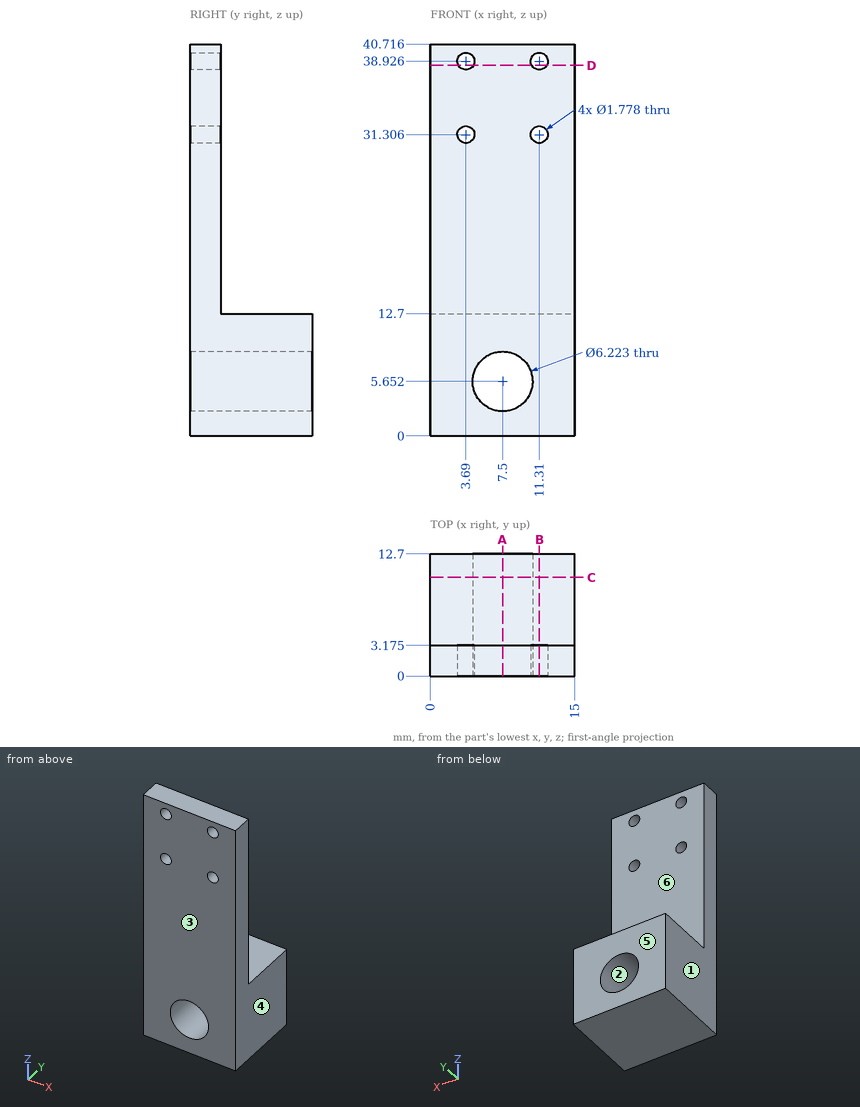
Design review of the part shown in the three views and the two pictorial views. Dimensions are in mm from the part's minimum x, y and z. A direction names the side the tool comes from. Coordinates: 2 decimals unless noted, no trailing zeros. Loops run counter-clockwise (first coordinate to the right, second up) from the corner with the lowest first, then second, coordinate; pieces in that order, holes last. Notation, with made-up numbers: M 26.5,6 L 78.5,6 A27 ccw 78.5,35 Z; hole C 26.5,45 d6. An arc over 180 degrees is marked long. One line per question, with ' | ' between items.
(1) We need section D-D (z = 38.5). Give the boundary of the cut face in (x, y) (1 decimal).
Filled in:
outline: M 0,0 L 2.9,0 L 2.9,3.2 L 0,3.2 Z; M 4.5,0 L 10.5,0 L 10.5,3.2 L 4.5,3.2 Z; M 12.1,0 L 15,0 L 15,3.2 L 12.1,3.2 Z
(2) We need section A-A (x = 7.5). Give the boundary of the cut face in (y, z) (1 decimal), and give its area (3 significant figures).
Filled in:
outline: M 0,0 L 12.7,0 L 12.7,2.5 L 0,2.5 Z; M 0,8.8 L 12.7,8.8 L 12.7,12.7 L 3.2,12.7 L 3.2,40.7 L 0,40.7 Z | area: 171 mm^2
(3) We need section B-B (x = 11.31). Give the boundary of the cut face in (y, z) (1 decimal).
Filled in:
outline: M 0,0 L 12.7,0 L 12.7,12.7 L 3.2,12.7 L 3.2,30.4 L 0,30.4 Z; M 0,32.2 L 3.2,32.2 L 3.2,38 L 0,38 Z; M 0,39.8 L 3.2,39.8 L 3.2,40.7 L 0,40.7 Z
(4) Draft analysis for pull direction X (two halves, no side actions). For the marked faces 1, 2, 3 and 4, state which applies: released by +X, released by -X, zero draft, split by the parting line, or undercut.
Filled in:
face 1: released by -X | face 2: undercut | face 3: zero draft | face 4: released by +X
(5) For pin 1 Ø1.1 at (x, z) = (3.69, 31.31) entering from +Y; pin 2 Ø1.5 at (x, y) = (10.5, 5.5) entering from +Z; pin 3 Ø8 at (x, z) = (8, 29.5) entering from +Y (1 decimal), all flat-tipped, find the tip position at first contact; note any pin that passes through.
Filled in:
pin 1: passes through | pin 2: stops at z = 12.7 | pin 3: stops at y = 3.2
(6) We need section C-C (y = 10.25). Give the boundary of the cut face in (x, z).
Filled in:
outline: M 0,0 L 15,0 L 15,12.7 L 0,12.7 Z; hole C 7.5,5.65 d6.22
(7) Wall thickness on probe 1 along Z at (x, y) = (12.5, 9); probe 2 along Z at (x, y) = (9.5, 9.25) (1 decimal); probe 3 along Y at (x, z) = (1, 32) (1 decimal): over which ranges is each line inside the solid? List them lowest first.
Filled in:
probe 1: z = 0 to 12.7 | probe 2: z = 0 to 3.3, 8 to 12.7 | probe 3: y = 0 to 3.2
(8) Machinability: for the marked faces 5 and 6, which of the approach directions +Z, -Z, +X, -X, +Y, -Y give a long, thin tool a straight path to every point of the face, cutting with its end or side? Answer none if there is none.
Filled in:
face 5: +Z, -Z, +X, -X, +Y | face 6: +Z, +X, -X, +Y
